```python
from build123d import *

# Parameters (mm, degrees)
FILLET1_R    = 101.6
SCALE1_SCALE = 0.214285714


with BuildPart() as part:
    # Sketch2 → Revolve1 (revolve)
    with BuildSketch(Plane.XY, mode=Mode.PRIVATE) as revolve1_sk:
        Polygon((0, 0), (304.8, 0), (304.8, -50.8), (254, -50.8), (254, -406.4), (304.8, -406.4), (304.8, -457.2), (0, -457.2), align=None)
    revolve(revolve1_sk.sketch.rotate(Axis((0, -457.2, 0), (0, 1, 0)), 90), axis=Axis((0, -457.2, 0), (0, 1, 0)))

    # Fillet1
    # the kernel refuses this fillet: 101.6 mm, written as the material it takes off along each edge
    with BuildSketch(Plane(origin=(0, -457.2, 0), x_dir=(0, 0, -1), z_dir=(1, 0, 0))) as fillet1_piece_1:
        with BuildLine():
            CenterArc((216.811818975, 101.6), FILLET1_R, 270, 60)
            Line((216.811818975, 0), (216.811818975, -2.032))
            Line((216.811818975, -2.032), (304.8, -2.032))
            Line((304.8, -2.032), (306.832, 0))
            ThreePointArc((306.832, 0), (306.832, 25.4), (306.55976362, 49.784))
            Line((306.55976362, 49.784), (304.8, 50.8))
        make_face()
    revolve(axis=Axis((0, -457.2, 0), (0, 1, 0)), mode=Mode.SUBTRACT)
    with BuildSketch(Plane(origin=(0, 0, 0), x_dir=(0, 0, -1), z_dir=(1, 0, 0))) as fillet1_piece_2:
        with BuildLine():
            CenterArc((216.811818975, -101.6), FILLET1_R, 30, 60)
            Line((304.8, -50.8), (306.55976362, -49.784))
            ThreePointArc((306.55976362, -49.784), (306.832, -25.4), (306.832, 0))
            Line((306.832, 0), (304.8, 2.032))
            Line((304.8, 2.032), (216.811818975, 2.032))
            Line((216.811818975, 2.032), (216.811818975, 0))
        make_face()
    revolve(axis=Axis((0, 0, 0), (0, 1, 0)), mode=Mode.SUBTRACT)


with BuildPart() as part_1:
    # Scale1: scaled about (0, -228.6, 0)
    add(part.part.scale(SCALE1_SCALE).moved(Location((0, -179.614285714, 0))))


solid = part_1.part
```
For this review, take the finished solid that the model builds, in its own axes (mm). Give positions to 0.01 mm unless a question says otherwise; leave off trailing zeros. Write each loop counter-clockwise with the first axis right and the second up, starting at its lowest first coordinate (ties: lowest second). Pieces come first, ordered by that corner, then holes. Notation, with made-up numbers: M 11.5,88 L 44.5,88 A15 ccw 44.5,109 Z; hole C 61,35 d5. An arc over 180 degrees is marked long. One line per item, written item: value.
1) The part is to be moulded in two halves that separate along Y. For faces 1 (the flat face through (-54, -266.7, -15)), 2 (the flat face through (-1, -179.614, -1)), 3 (the flat face through (-1, -277.586, 1)), say which applies: +Y half, -Y half, draft (parallel to the pull), parting line (faces both ways), or undercut.
Results are:
face 1: undercut
face 2: +Y half
face 3: -Y half
2) For P1, Ø10, axis at x = -4.5, y = -247, coming from the -Z side; P2, Ø8, axis at x = 13, y = -247, coming from the +Z side; P3, Ø5, axis at x = -39.5, y = -236.5, coming from the +Z side, all flat-tipped, find the tip position at first contact; note any pin that passes through.
Results are:
P1: stops at z = -54.43
P2: stops at z = 53.68
P3: stops at z = 39.92
3) Take a section at C-C, the plane y = -204. Write out the cut boundary in (x, z).
Results are:
outline: C 0,0 d108.86
4) Take a section at B-B, the plane x = 0. Write out the cut boundary in (y, z).
Results are:
outline: M -277.59,-46.46 A21.77 ccw -266.7,-65.31 L -266.7,-54.43 L -190.5,-54.43 L -190.5,-65.31 A21.77 ccw -179.61,-46.46 L -179.61,46.46 A21.77 ccw -190.5,65.31 L -190.5,54.43 L -266.7,54.43 L -266.7,65.31 A21.77 ccw -277.59,46.46 Z
5) Take a section at A-A, the plane z = 0. Write out the cut boundary in (x, y).
Results are:
outline: M -65.31,-266.7 A21.77 ccw -46.46,-277.59 L 46.46,-277.59 A21.77 ccw 65.31,-266.7 L 54.43,-266.7 L 54.43,-190.5 L 65.31,-190.5 A21.77 ccw 46.46,-179.61 L -46.46,-179.61 A21.77 ccw -65.31,-190.5 L -54.43,-190.5 L -54.43,-266.7 Z
6) For line 1 (Y direction, x = 59, z = 19); line 2 (X direction, y = -195.5, z = 20); line 3 (Z direction, x = -16, y = -262.5), list the stretches that pass through material, from the lowest coordinate up. Write a range as from..to.
Results are:
line 1: y = -271.08..-266.7, -190.5..-186.12
line 2: x = -50.62..50.62
line 3: z = -52.02..52.02
